CAD build for the part. Positions are in the model's coordinates, mm. Face numbers are marked on the shaded views. A direction names the side the tool comes from. Give positions to 0.01 mm unless a question says otherwise; leave off trailing zeros. Write each loop counter-clockwise with the first axis right and the second up, starting at its lowest first coordinate (ties: lowest second). Pieces come first, ordered by that corner, then holes. Notation, with made-up numbers: (-28.75, 3.5) - (-21.75, 3.5) arc R7 ccw to (-21.75, 13.5) - close; hole circle Ø9 at (-38, 89.25). An arc over 180 degrees is marked (long way). Answer as a JSON object with one key per item and string values.
from build123d import *

# Parameters (mm, degrees)
ESQUISSE1_W             = 70
ESQUISSE1_H             = 41
BOSS_EXTRU_1_DEPTH      = 22
COQUE1_T                = -2
BOSS_EXTRU_2_DEPTH      = 10
ENL_V_MAT_EXTRU_1_REACH = 76.352
ESQUISSE3_R             = 4
ESQUISSE3_W             = 8
ESQUISSE3_H             = 4
ENL_V_MAT_EXTRU_2_REACH = 76.352
ESQUISSE4_R             = 3.5
CONG_1_R                = 1
CHANFREIN1_SIZE         = 2


with BuildPart() as part:
    # Esquisse1 → Boss.-Extru.1 (new body)
    with BuildSketch(Plane(origin=(0, 0, 0), x_dir=(1, 0, 0), z_dir=(0, 1, 0))):
        Rectangle(ESQUISSE1_W, ESQUISSE1_H)
    extrude(amount=BOSS_EXTRU_1_DEPTH)

    # Coque1
    coque1_openings = [part.faces().sort_by_distance(p)[0] for p in [
        (0, 22, 0),
    ]]
    offset(amount=COQUE1_T, openings=coque1_openings, kind=Kind.INTERSECTION)

    # Esquisse2 → Boss.-Extru.2 (add)
    with BuildSketch(Plane(origin=(0, 2, 0), x_dir=(1, 0, 0), z_dir=(0, 1, 0))):
        Polygon((33, -16.5), (24, -16.5), (11.5, -18.5), (33, -18.5), align=None)
        Polygon((33, -6.2), (24, -6.2), (11.5, -4.2), (2, -4.2), (2, -1.5), (33, -1.5), align=None)
    extrude(amount=BOSS_EXTRU_2_DEPTH)

    # Esquisse3 → Enlèv. mat.-Extru.1 (cut, up to next)
    with BuildSketch(Plane.ZY.offset(-33), mode=Mode.PRIVATE) as enl_v_mat_extru_1_sk1:
        with Locations((11.35, 7.5)):
            Circle(ESQUISSE3_R)
    enl_v_mat_extru_1_tool1 = extrude(enl_v_mat_extru_1_sk1.sketch, amount=-ENL_V_MAT_EXTRU_1_REACH, mode=Mode.PRIVATE) & part.part
    # Esquisse3 → Enlèv. mat.-Extru.1 (cut, up to next)
    with BuildSketch(Plane.ZY.offset(-33), mode=Mode.PRIVATE) as enl_v_mat_extru_1_sk2:
        with Locations((-8.5, 8.5)):
            Rectangle(ESQUISSE3_W, ESQUISSE3_H)
    enl_v_mat_extru_1_tool2 = extrude(enl_v_mat_extru_1_sk2.sketch, amount=-ENL_V_MAT_EXTRU_1_REACH, mode=Mode.PRIVATE) & part.part
    add(enl_v_mat_extru_1_tool1.solids().sort_by_distance((33, 7.5, 11.35))[0], mode=Mode.SUBTRACT)
    add(enl_v_mat_extru_1_tool2.solids().sort_by_distance((33, 8.5, -8.5))[0], mode=Mode.SUBTRACT)

    # Esquisse4 → Enlèv. mat.-Extru.2 (cut, up to next)
    with BuildSketch(Plane(origin=(-33, 0, 0), x_dir=(0, 0, -1), z_dir=(1, 0, 0)), mode=Mode.PRIVATE) as enl_v_mat_extru_2_sk1:
        with Locations((-11.35, 7.5)):
            Circle(ESQUISSE4_R)
    enl_v_mat_extru_2_tool1 = extrude(enl_v_mat_extru_2_sk1.sketch, amount=-ENL_V_MAT_EXTRU_2_REACH, mode=Mode.PRIVATE) & part.part
    add(enl_v_mat_extru_2_tool1.solids().sort_by_distance((-33, 7.5, 11.35))[0], mode=Mode.SUBTRACT)

    # Congé1
    cong_1_edges = [part.edges().sort_by_distance(p)[0] for p in [
        (33, 17, 18.5),
        (0, 2, -18.5),
        (33, 12, -18.5),
        (-33, 2, 0),
        (-33, 12, -18.5),
        (-10.75, 2, 18.5),
        (-33, 12, 18.5),
        (33, 2, 11.35),
        (28.5, 2, 16.5),
        (33, 7, 16.5),
        (17.75, 2, 17.5),
        (33, 12, 17.5),
        (22.25, 12, 18.5),
        (33, 2, -8.5),
        (33, 7, 6.2),
        (17.5, 2, 1.5),
        (33, 7, 1.5),
        (2, 2, 2.85),
        (2, 7, 1.5),
        (6.75, 2, 4.2),
        (2, 7, 4.2),
        (17.75, 2, 5.2),
        (28.5, 2, 6.2),
        (33, 12, 3.85),
        (17.5, 12, 1.5),
        (2, 12, 2.85),
        (6.75, 12, 4.2),
        (17.75, 12, 5.2),
        (28.5, 12, 6.2),
    ]]
    fillet(cong_1_edges, radius=CONG_1_R)

    # Chanfrein1
    chanfrein1_edges = [part.edges().sort_by_distance(p)[0] for p in [
        (0, 0, 20.5),
        (-35, 0, 0),
        (0, 0, -20.5),
        (35, 0, 0),
        (35, 11, 20.5),
        (-35, 11, 20.5),
        (-35, 11, -20.5),
        (35, 11, -20.5),
    ]]
    chamfer(chanfrein1_edges, length=CHANFREIN1_SIZE)


solid = part.part
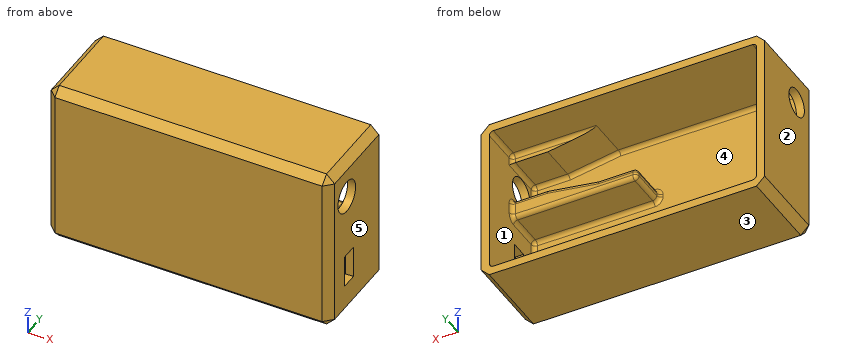
(1) 3-axis set-ups, long thin cutter, end or side, ignore diameter. For the marked faces 1 and 2: which of +Z, -Z, +X, -X, +Y, -Y reach the whole face in a straight line?
Answer key:
{"face 1": "+Y", "face 2": "+Z, -Z, -X, +Y, -Y"}
(2) Saw through at D-D, the plane z = -3. Give the cut face in (x, y).
Answer key:
{"outline": "(-35, 2) - (-33, 0) - (33, 0) - (35, 2) - (35, 22) - (33, 22) - (33, 3) arc R1 cw to (32, 2) - (-32, 2) arc R1 cw to (-33, 3) - (-33, 22) - (-35, 22) - close"}
(3) Flat gauge pins, fed straight in: P1, Ø12, axis at x = -7.5, z = 11, coming from the +Y side; P2, Ø1.4, axis at x = 20.5, z = 4, coming from the +Y side; P3, Ø1.6, axis at x = 34.5, y = 8.5, coming from the -Z side. Where does each tip first touch, or does it go through?
Answer key:
{"P1": "stops at y = 2", "P2": "stops at y = 12", "P3": "stops at z = -19.8"}
(4) Pull direction X, two halves, no side cores. Call the marked faces 3, 4 and 5: pulls with the +X half, pulls with the -X half, needs draft (parallel to the pull), parting line crosses it, or undercut.
Answer key:
{"face 3": "needs draft", "face 4": "undercut", "face 5": "pulls with the +X half"}
(5) Saw through at A-A, the plane z = 11.35. Give the cut face in (x, y), and give its area (3 significant figures).
Answer key:
{"outline": "(-35, 2) - (-33, 0) - (33, 0) - (35, 2) - (35, 3.5) - (33, 3.5) - (33, 3) arc R1 cw to (32, 2) - (-32, 2) arc R1 cw to (-33, 3) - (-33, 4) - (-35, 4) - close; (-35, 11) - (-33, 11) - (-33, 22) - (-35, 22) - close; (33, 11.5) - (35, 11.5) - (35, 22) - (33, 22) - close", "area": "186 mm²"}
(6) Saw through at B-B, the plane y = 17.25. Give the cut face in (x, z), and give its area (3 significant figures).
Answer key:
{"outline": "(-35, -18.5) - (-33, -20.5) - (33, -20.5) - (35, -18.5) - (35, 18.5) - (33, 20.5) - (-33, 20.5) - (-35, 18.5) - close; hole (-33, -17.5) arc R1 ccw to (-32, -18.5) - (32, -18.5) arc R1 ccw to (33, -17.5) - (33, 17.5) arc R1 ccw to (32, 18.5) - (-32, 18.5) arc R1 ccw to (-33, 17.5) - close", "area": "421 mm²"}
(7) Probe L1, parallel to X at y = 12.5, z = -13; L2, parallel to Z at x = -6.5, y = 21; L3, parallel to Y at x = -33.5, z = 11.35. List the from-to ranges inside material, lowest first. Write a range as [from, to].
Answer key:
{"L1": "x = [-35, -33], [33, 35]", "L2": "z = [-20.5, -18.5], [18.5, 20.5]", "L3": "y = [0.5, 4], [11, 22]"}
(8) Saw through at C-C, the plane x = 27. Give the cut face in (y, z).
Answer key:
{"outline": "(0, -18.5) - (2, -20.5) - (22, -20.5) - (22, -18.5) - (3, -18.5) arc R1 cw to (2, -17.5) - (2, 0.5) arc R1 cw to (3, 1.5) - (11, 1.5) arc R1 ccw to (12, 2.5) - (12, 5.2) arc R1 ccw to (11, 6.2) - (3, 6.2) arc R1 cw to (2, 7.2) - (2, 15.5) arc R1 cw to (3, 16.5) - (12, 16.5) - (12, 17.5) arc R1 cw to (13, 18.5) - (22, 18.5) - (22, 20.5) - (2, 20.5) - (0, 18.5) - close"}
